from build123d import *

# Parameters (mm, degrees)
F0_R     = 2.5
F1_DEPTH = 2
F2_R     = 0.5
F3_SIZE  = 0.5


with BuildPart() as f1:
    # F0 (on Front) → F1 (new body)
    with BuildSketch(Plane.XZ):
        with BuildLine():
            Line((10.5747856316, 13.0727361555), (-16.4252143684, 13.0727361555))
            ThreePointArc((-16.4252143684, 13.0727361555), (-22.9252143684, 6.5727361555), (-16.4252143684, 0.0727361555))
            Line((-16.4252143684, 0.0727361555), (10.5747856316, 0.0727361555))
            ThreePointArc((10.5747856316, 0.0727361555), (17.0747856316, 6.5727361555), (10.5747856316, 13.0727361555))
        make_face()
        with Locations((10.5747856316, 6.5727361555)):
            Circle(F0_R, mode=Mode.SUBTRACT)
        with Locations((-16.4252143684, 6.5727361555)):
            Circle(F0_R, mode=Mode.SUBTRACT)
    extrude(amount=F1_DEPTH)

    # F2
    f2_edges = [f1.edges().sort_by_distance(p)[0] for p in [
        (-22.925214, -2, 6.572736),
        (-2.925214, 0, 0.072736),
    ]]
    fillet(f2_edges, radius=F2_R)

    # F3
    f3_edges = [f1.edges().sort_by_distance(p)[0] for p in [
        (-18.925214, -2, 6.572736),
        (8.074786, 0, 6.572736),
        (8.074786, -2, 6.572736),
        (-2.925214, -0.5, 13.072736),
        (-18.925214, 0, 6.572736),
    ]]
    chamfer(f3_edges, length=F3_SIZE)


solid = f1.part
The listing builds one solid part. Answer for the finished solid, in the listing's coordinates (mm). Round coordinates to 2 decimals unless told otherwise and drop trailing zeros. Loops run counter-clockwise (first coordinate to the right, second up) from the corner with the lowest first, then second, coordinate; pieces in that order, holes last. Notation, with made-up numbers: M 10.25,19 L 18.25,19 A30 cw 18.25,42 Z; hole C 86.5,-27 d1. An arc over 180 degrees is marked long. Return JSON: item names as keys, results as strings.
Q1. Find section A-A, the plane y = -1.15. Determine the outline of the cut face in (x, z).
Results list:
{"outline": "M -16.43,0.07 L 10.57,0.07 A6.5 ccw 10.57,13.07 L -16.43,13.07 A6.5 ccw Z; hole C -16.43,6.57 d5; hole C 10.57,6.57 d5"}
Q2. Find the intervals of material crossed by line 1 along X through (y, z) = (-0.55, 6); line 2 along X through (y, z) = (-1.85, 8.75); line 3 along Z through (x, y) = (12.5, -1.4), in increasing order. Write a range as from..to.
Results list:
{"line 1": "x = -22.9..-18.86, -13.99..8.14, 13.01..17.05", "line 2": "x = -22.4..-18.26, -14.59..8.74, 12.41..16.55", "line 3": "z = 0.36..4.98, 8.17..12.78"}
Q3. Find section B-B, the plane z = 5.5. State how many separate pieces and enclosed holes the cut face has, plus the area to 3 significant figures.
Results list:
{"separate pieces": "3", "enclosed holes": "0", "area": "60.3 mm2"}
Q4. The mould has two halves that part along Z. Classify faces 1 (the face through (17.073, -0.993, 6.43)), 2 (the face through (8.077, -0.993, 6.683)), 3 (the face through (-3, 0, 7)): released by +Z, released by -Z, zero draft, split by the parting line, or undercut.
Results list:
{"face 1": "split by the parting line", "face 2": "undercut", "face 3": "zero draft"}
